Geometry: final body of the model. Coordinates: model frame, mm. Face numbers are marked on the shaded views. A direction names the side the tool comes from. Give positions to 0.01 mm unless a question says otherwise; leave off trailing zeros. Write each loop counter-clockwise with the first axis right and the second up, starting at its lowest first coordinate (ties: lowest second). Pieces come first, ordered by that corner, then holes.
Q1. Section C-C (x = 3.25). Return the cut outline in (y, z), plus the area to 4 significant figures.
Q2. Line query: line 1 (X direction, y = 2.25, z = -15); line 2 (Z direction, x = 3.5, y = 9.5); line 3 (Z direction, x = 1.5, y = 8.75). Output: solid intervals per line, ascending.
Q3. Section D-D (z = -9). Return the cut outline in (x, y), plus the area to 3 significant figures.
Q4. Reachability of the marked faces 4, 5, 6 and 7 from +Z, -Z, +X, -X, +Y, -Y: full face, straight path, thin tool, end or side. Return the list, or none.
Q5. Section B-B (z = -15). Return the cut outline in (x, y), plus the area to 3 significant figures.
Q6. Mould query, pull axis Z, two halves, no side actions, for the marked faces 1, 2 and 3. Classes: +Z half, -Z half, draft (parallel to the pull), parting line (faces both ways), or undercut.
Q7. Section A-A (y = 1.75). Return the cut outline in (x, z).
Q8. Pin query (flat end, axial travel): pin 1 Ø5 at (y, z) = (1.5, -4.5) entering from +X; pin 2 Ø3.5 at (y, z) = (2.5, -15) entering from -X; pin 3 Ø1.7 at (x, y) = (1, 10) entering from -Z; pin 4 Ø2.5 at (y, z) = (2, -15) entering from +X. Return the tip coordinate at first contact, or that it passes through.
from build123d import *

# Parameters (mm, degrees)
BOSS_EXTRUDE1_DEPTH = 0.5
SKETCH2_W           = 8
SKETCH2_H           = 0.5
BOSS_EXTRUDE2_DEPTH = 14
BOSS_EXTRUDE3_DEPTH = 3
SKETCH4_R           = 1.5
CUT_EXTRUDE1_DEPTH  = 13
FILLET1_R           = 0.5
FILLET2_R           = 0.5
SKETCH5_R           = 2.838371804
BOSS_EXTRUDE4_DEPTH = 0.3


with BuildPart() as part:
    # Sketch1 → Boss-Extrude1 (new body)
    with BuildSketch(Plane(origin=(0, 0, 0), x_dir=(1, 0, 0), z_dir=(0, 1, 0))):
        Polygon((0, 0), (-4, 0), (-4, 18), (4, 18), (4, 0), align=None)
    extrude(amount=BOSS_EXTRUDE1_DEPTH)

    # Sketch2 → Boss-Extrude2 (add)
    with BuildSketch(Plane(origin=(0, 0, 0), x_dir=(1, 0, 0), z_dir=(0, 1, 0))):
        with Locations((0, 0.25)):
            Rectangle(SKETCH2_W, SKETCH2_H)
    extrude(amount=BOSS_EXTRUDE2_DEPTH)

    # Sketch3 → Boss-Extrude3 (add)
    with BuildSketch(Plane(origin=(0, 0.5, 0), x_dir=(1, 0, 0), z_dir=(0, 1, 0))):
        Polygon((0, 18), (-2.598076211, 16.5), (-2.598076211, 13.5), (0, 12), (2.598076211, 13.5), (2.598076211, 16.5), align=None)
    extrude(amount=BOSS_EXTRUDE3_DEPTH)

    # Sketch4 → Cut-Extrude1 (cut)
    with BuildSketch(Plane(origin=(0, 3.5, 0), x_dir=(1, 0, 0), z_dir=(0, 1, 0))):
        with Locations(Location((0, 15, 0), (0, 0, 270))):
            Circle(SKETCH4_R)
    extrude(amount=-CUT_EXTRUDE1_DEPTH, mode=Mode.SUBTRACT)

    # Fillet1
    fillet1_edges = [part.edges().sort_by_distance(p)[0] for p in [
        (0, 0, 0),
    ]]
    fillet(fillet1_edges, radius=FILLET1_R)

    # Fillet2
    fillet2_edges = [part.edges().sort_by_distance(p)[0] for p in [
        (0, 0.5, -0.5),
    ]]
    fillet(fillet2_edges, radius=FILLET2_R)

    # Sketch5 → Boss-Extrude4 (add)
    with BuildSketch(Plane(origin=(0, 0, -0.5), x_dir=(-1, 0, 0), z_dir=(0, 0, -1))):
        with Locations(Location((0, 10.341282462, 0), (0, 0, 180))):
            Circle(SKETCH5_R)
    extrude(amount=BOSS_EXTRUDE4_DEPTH)


solid = part.part
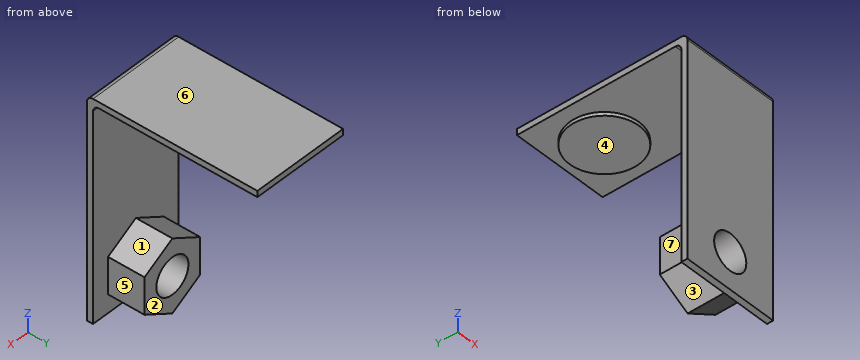
Computed:
1. outline: (0, -18) - (0.5, -18) - (0.5, -1) arc R0.5 cw to (1, -0.5) - (14, -0.5) - (14, 0) - (0.5, 0) arc R0.5 ccw to (0, -0.5) - close
1. area: 15.75 mm2
2. line 1: x = -2.6 to -1.5, 1.5 to 2.6
2. line 2: z = -0.5 to 0
2. line 3: z = -0.8 to 0
3. outline: (-4, 0) - (4, 0) - (4, 0.5) - (-4, 0.5) - close
3. area: 4.00 mm2
4. face 4: -Z, +X, -X, +Y
4. face 5: -Z, +X, +Y
4. face 6: +Z, +X, -X, +Y, -Y
4. face 7: -Z, -X, +Y
5. outline: (-4, 0) - (-1.5, 0) - (-1.5, 3.5) - (-2.6, 3.5) - (-2.6, 0.5) - (-4, 0.5) - close; (1.5, 0) - (4, 0) - (4, 0.5) - (2.6, 0.5) - (2.6, 3.5) - (1.5, 3.5) - close
5. area: 9.09 mm2
6. face 1: undercut
6. face 2: draft
6. face 3: -Z half
7. outline: (-4, -0.5) - (4, -0.5) - (4, 0) - (-4, 0) - close; (-2.6, -16.5) - (0, -18) - (2.6, -16.5) - (2.6, -13.5) - (0, -12) - (-2.6, -13.5) - close; hole circle Ø3 at (0, -15)
8. pin 1: stops at x = 4
8. pin 2: stops at x = -2.6
8. pin 3: stops at z = -0.8
8. pin 4: stops at x = 2.6
